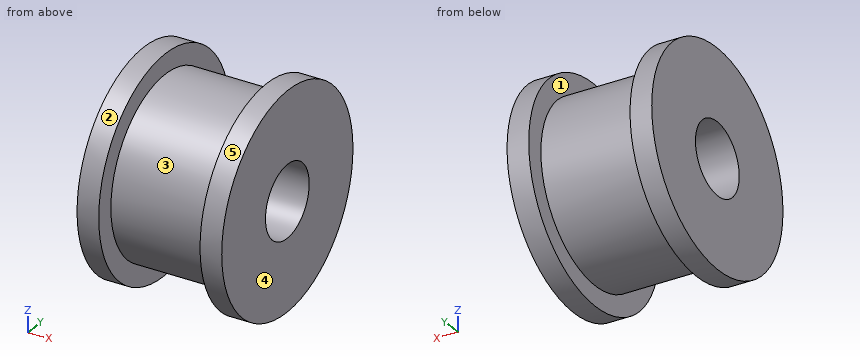
Autodesk Fusion 360 part; units mm, degrees
sketch "Sketch1" plane through (0, 0, 0) normal (1, 0, 0) x (0, 1, 0)
  circle A0 centre (0, 0) radius 6.11
  circle A1 centre (0, 0) radius 7.5
  circle A2 centre (0, 0) radius 2.5
  circle A3 centre (0, 0) radius 6.365 construction
  dimension "d1" = 5
  dimension "d2" = 12.22
  dimension "d3" = 15
  dimension "d11" = 12.73
extrude "Extrude1" add sketch "Sketch1" along normal blind 10 contours A0 | A1
extrude "Extrude2" cut sketch "Sketch1" along normal blind 7 from surface at 1.5 contours A1
equation "d2 = outside_dia"
equation "pitch_dia = 12.73 mm"
equation "outside_dia = 12.22 mm"
equation "d11 = pitch_dia"
The model under review builds one solid part; all positions refer to its coordinate system, in mm. Face numbers are marked on the shaded views. A direction names the side the tool comes from. Round coordinates to 2 decimals unless told otherwise and drop trailing zeros. Order: outer loops, then holes, each group sorted by start corner. A loop starts at its lowest first (then second) coordinate and runs counter-clockwise, first axis right, second up. Notation, with made-up numbers: (34, 7) -> (75, 7) arc R27 cw to (75, 38) -> close; hole circle Ø5 at (70.25, 56.5). An arc over 180 degrees is marked (long way). Use a Markdown table: item, result.
Q1. Mouldability with a two-part tool opening along X and no side actions: class the marked faces 3, 4 and 5 as +X half, -X half, draft (parallel to the pull), parting line (faces both ways), or undercut.
Values:
| item | result |
|---|---|
| face 3 | undercut |
| face 4 | +X half |
| face 5 | draft |
Q2. We need section C-C on x = 9. Write out the cut boundary in (y, z).
Values:
| item | result |
|---|---|
| outline | circle Ø15 at (0, 0); hole circle Ø5 at (0, 0) |
Q3. We need section D-D on z = 3.25. Write out the cut boundary in (x, y), then the cut area to 3 significant figures.
Values:
| item | result |
|---|---|
| outline | (0, -6.76) -> (1.5, -6.76) -> (1.5, -5.17) -> (8.5, -5.17) -> (8.5, -6.76) -> (10, -6.76) -> (10, 6.76) -> (8.5, 6.76) -> (8.5, 5.17) -> (1.5, 5.17) -> (1.5, 6.76) -> (0, 6.76) -> close |
| area | 113 mm^2 |
Q4. Clearance check with flat-ended pins moving along their axes: P1, Ø2, axis at y = -0.5, z = 1, coming from the -X side; P2, Ø5, axis at x = 2.5, z = -6, coming from the +Y side; P3, Ø1.5, axis at x = 5, z = 1.5, coming from the +Y side; P4, Ø4, axis at x = 4.5, y = -6, coming from the +Z side. State where each tip first meets the part, or that it passes through.
Values:
| item | result |
|---|---|
| P1 | passes through |
| P2 | stops at y = 6.52 |
| P3 | stops at y = 6.06 |
| P4 | stops at z = 4.62 |
Q5. We need section A-A on z = 0. Write out the cut boundary in (x, y), then the cut area to 3 significant figures.
Values:
| item | result |
|---|---|
| outline | (0, -7.5) -> (1.5, -7.5) -> (1.5, -6.11) -> (8.5, -6.11) -> (8.5, -7.5) -> (10, -7.5) -> (10, -2.5) -> (0, -2.5) -> close; (0, 2.5) -> (10, 2.5) -> (10, 7.5) -> (8.5, 7.5) -> (8.5, 6.11) -> (1.5, 6.11) -> (1.5, 7.5) -> (0, 7.5) -> close |
| area | 80.5 mm^2 |
Q6. Tool access review of the marked faces 1 and 2: name each direction out of +Z, -Z, +X, -X, +Y, -Y from which nothing blocks a thin tool from reaching the whole face with its end or side.
Values:
| item | result |
|---|---|
| face 1 | none |
| face 2 | +X, -X |
Q7. For line 1 (X direction, y = 3, z = -6.25); line 2 (Z direction, x = 5, y = 0); line 3 (Y direction, x = 3.75, z = -2), list the stretches that pass through material, from the lowest coordinate up.
Values:
| item | result |
|---|---|
| line 1 | x = 0 to 1.5, 8.5 to 10 |
| line 2 | z = -6.11 to -2.5, 2.5 to 6.11 |
| line 3 | y = -5.77 to -1.5, 1.5 to 5.77 |
